Could you check a few things on this model? Use its own coordinates, in mm. Face numbers are marked on the shaded views. A direction names the side the tool comes from. Coordinates: 2 decimals unless noted, no trailing zeros. Write each loop counter-clockwise with the first axis right and the second up, starting at its lowest first coordinate (ties: lowest second). Pieces come first, ordered by that corner, then holes. Notation, with made-up numbers: M 23.5,39.5 L 55.5,39.5 A22 ccw 55.5,47.5 Z; hole C 9,79 d10. An arc over 180 degrees is marked long. Write item = value, one per line.
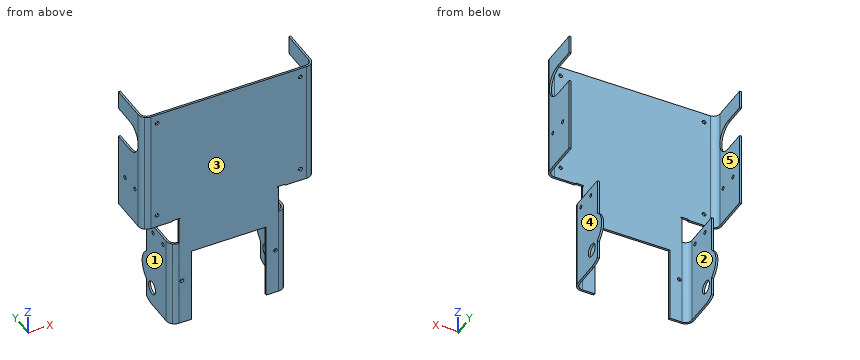
```python
from build123d import *

# Parameters (mm, degrees)
BOSS_EXTRUDE2_DEPTH     = 1.6
EDGE_FLANGE1_START      = -50
EDGE_FLANGE1_DEPTH      = 100
EDGE_FLANGE1_START_2    = -143
EDGE_FLANGE1_2_DEPTH    = 93.8
EDGE_FLANGE1_3_DEPTH    = 0.8
EDGE_FLANGE1_4_DEPTH    = 100
EDGE_FLANGE1_5_DEPTH    = 93
CUT_EXTRUDE1_START      = -71.5
CUT_EXTRUDE1_DEPTH      = 21.5
SKETCH24_R              = 15
BOSS_EXTRUDE3_DEPTH     = 1.6
BOSS_EXTRUDE4_START     = -1.6
SKETCH25_R              = 15
BOSS_EXTRUDE4_DEPTH     = 1.6
SKETCH26_R              = 5.25
CUT_EXTRUDE2_DEPTH      = 109.6
CUT_EXTRUDE3_DEPTH      = 1000
CUT_EXTRUDE4_DEPTH      = 188.95057861
CUT_EXTRUDE4_DEPTH_BACK = 188.95057861
SKETCH30_R              = 1.5
CUT_EXTRUDE5_DEPTH      = 204.484274577
CUT_EXTRUDE5_DEPTH_BACK = 204.484274577
SKETCH32_R              = 1.5
CUT_EXTRUDE6_DEPTH      = 54


# Read off the part's stored shape, not the designer's step: Edge-Flange1, Cut-Extrude1
with BuildPart() as part:
    # Sketch1 → Boss-Extrude2 (new body)
    with BuildSketch(Plane(origin=(0, 0, 0), x_dir=(1, 0, 0), z_dir=(0, 1, 0))):
        Polygon((45, 50), (45, 143), (30, 143), (30, 82), (-30, 82), (-30, 143), (-45, 143), (-45, 50), (-67.5, 50), (-67.5, -50), (67.5, -50), (67.5, 50), align=None)
    extrude(amount=BOSS_EXTRUDE2_DEPTH)

    # Edge-Flange1 outline → Edge-Flange1 (cut)
    with BuildSketch(Plane.XY.offset(EDGE_FLANGE1_START)):
        with BuildLine():
            Line((-67.5, 0), (-62.5, 0))
            ThreePointArc((-62.5, 0), (-64.797825059, 0.412916681), (-66.808131846, 1.6))
            Line((-66.808131846, 1.6), (-67.5, 1.6))
            Line((-67.5, 1.6), (-67.5, 0))
        make_face()
        with BuildLine():
            ThreePointArc((66.808131846, 1.6), (64.797825059, 0.412916681), (62.5, 0))
            Line((62.5, 0), (67.5, 0))
            Line((67.5, 0), (67.5, 1.6))
            Line((67.5, 1.6), (66.808131846, 1.6))
        make_face()
    extrude(amount=EDGE_FLANGE1_DEPTH, mode=Mode.SUBTRACT)

    # Edge-Flange1 2 outline → Edge-Flange1 2 (cut)
    with BuildSketch(Plane.XY.offset(EDGE_FLANGE1_START_2)):
        with BuildLine():
            Line((-45, 1.6), (-45, 0))
            Line((-45, 0), (-40, 0))
            ThreePointArc((-40, 0), (-42.297825059, 0.412916681), (-44.308131846, 1.6))
            Line((-44.308131846, 1.6), (-45, 1.6))
        make_face()
        with BuildLine():
            ThreePointArc((44.308131846, 1.6), (42.297825059, 0.412916681), (40, 0))
            Line((40, 0), (45, 0))
            Line((45, 0), (45, 1.6))
            Line((45, 1.6), (44.308131846, 1.6))
        make_face()
    extrude(amount=EDGE_FLANGE1_2_DEPTH, mode=Mode.SUBTRACT)

    # Edge-Flange1 3 outline → Edge-Flange1 3 (cut)
    with BuildSketch(Plane.XY.offset(EDGE_FLANGE1_START)):
        with BuildLine():
            ThreePointArc((-44.308131846, 1.6), (-42.297825059, 0.412916681), (-40, 0))
            Line((-40, 0), (-39.2, 0))
            Line((-39.2, 0), (-39.2, 1.6))
            Line((-39.2, 1.6), (-44.308131846, 1.6))
        make_face()
        with BuildLine():
            Line((39.2, 1.6), (39.2, 0))
            Line((39.2, 0), (40, 0))
            ThreePointArc((40, 0), (42.297825059, 0.412916681), (44.308131846, 1.6))
            Line((44.308131846, 1.6), (39.2, 1.6))
        make_face()
    extrude(amount=EDGE_FLANGE1_3_DEPTH, mode=Mode.SUBTRACT)

    # Edge-Flange1 4 outline → Edge-Flange1 4 (add)
    with BuildSketch(Plane.XY.offset(EDGE_FLANGE1_START)):
        with BuildLine():
            Line((-66.808131846, 1.6), (-62.5, 1.6))
            ThreePointArc((-62.5, 1.6), (-66.035533906, 3.064466094), (-67.5, 6.6))
            Line((-67.5, 6.6), (-67.5, 36.6))
            Line((-67.5, 36.6), (-69.1, 36.6))
            Line((-69.1, 36.6), (-69.1, 6.6))
            ThreePointArc((-69.1, 6.6), (-68.499736252, 3.84987911), (-66.808131846, 1.6))
        make_face()
        with BuildLine():
            ThreePointArc((67.5, 6.6), (66.035533906, 3.064466094), (62.5, 1.6))
            Line((62.5, 1.6), (66.808131846, 1.6))
            ThreePointArc((66.808131846, 1.6), (68.499736252, 3.84987911), (69.1, 6.6))
            Line((69.1, 6.6), (69.1, 36.6))
            Line((69.1, 36.6), (67.5, 36.6))
            Line((67.5, 36.6), (67.5, 6.6))
        make_face()
    extrude(amount=EDGE_FLANGE1_4_DEPTH)

    # Edge-Flange1 5 outline → Edge-Flange1 5 (add)
    with BuildSketch(Plane.XY.offset(EDGE_FLANGE1_START_2)):
        with BuildLine():
            ThreePointArc((-46.6, 6.6), (-45.999736252, 3.84987911), (-44.308131846, 1.6))
            Line((-44.308131846, 1.6), (-40, 1.6))
            ThreePointArc((-40, 1.6), (-43.535533906, 3.064466094), (-45, 6.6))
            Line((-45, 6.6), (-45, 36.6))
            Line((-45, 36.6), (-46.6, 36.6))
            Line((-46.6, 36.6), (-46.6, 6.6))
        make_face()
        with BuildLine():
            ThreePointArc((45, 6.6), (43.535533906, 3.064466094), (40, 1.6))
            Line((40, 1.6), (44.308131846, 1.6))
            ThreePointArc((44.308131846, 1.6), (45.999736252, 3.84987911), (46.6, 6.6))
            Line((46.6, 6.6), (46.6, 36.6))
            Line((46.6, 36.6), (45, 36.6))
            Line((45, 36.6), (45, 6.6))
        make_face()
    extrude(amount=EDGE_FLANGE1_5_DEPTH)

    # Cut-Extrude1 outline → Cut-Extrude1 (cut)
    with BuildSketch(Plane.XY.offset(CUT_EXTRUDE1_START)):
        with BuildLine():
            ThreePointArc((45, 6.6), (43.535533906, 3.064466094), (40, 1.6))
            Line((40, 1.6), (40, 0))
            ThreePointArc((40, 0), (44.666904756, 1.933095244), (46.6, 6.6))
            Line((46.6, 6.6), (46.6, 36.6))
            Line((46.6, 36.6), (45, 36.6))
            Line((45, 36.6), (45, 6.6))
        make_face()
        with BuildLine():
            ThreePointArc((-46.6, 6.6), (-44.666904756, 1.933095244), (-40, 0))
            Line((-40, 0), (-40, 1.6))
            ThreePointArc((-40, 1.6), (-43.535533906, 3.064466094), (-45, 6.6))
            Line((-45, 6.6), (-45, 36.6))
            Line((-45, 36.6), (-46.6, 36.6))
            Line((-46.6, 36.6), (-46.6, 6.6))
        make_face()
    extrude(amount=CUT_EXTRUDE1_DEPTH, mode=Mode.SUBTRACT)

    # Sketch24 → Boss-Extrude3 (add)
    with BuildSketch(Plane(origin=(46.6, 0, 0), x_dir=(0, 0, -1), z_dir=(1, 0, 0))):
        with Locations((113.002063462, 28.1)):
            Circle(SKETCH24_R)
    extrude(amount=-BOSS_EXTRUDE3_DEPTH)

    # Sketch25 → Boss-Extrude4 (add)
    with BuildSketch(Plane.ZY.offset(46.6).offset(BOSS_EXTRUDE4_START)):
        with Locations((-113.002063462, 28.1)):
            Circle(SKETCH25_R)
    extrude(amount=BOSS_EXTRUDE4_DEPTH)

    # Sketch26 → Cut-Extrude2 (cut)
    with BuildSketch(Plane(origin=(46.6, 0, 0), x_dir=(0, 0, -1), z_dir=(1, 0, 0))):
        with Locations(Location((128.002063462, 28.1, 0), (0, 0, 90))):
            Circle(SKETCH26_R)
        with BuildLine():
            Line((140.361270556, 36.6), (143, 36.6))
            Line((143, 36.6), (143, 28.348796314))
            ThreePointArc((143, 28.348796314), (142.289257641, 32.669035183), (140.361270556, 36.6))
        make_face()
    extrude(amount=-CUT_EXTRUDE2_DEPTH, mode=Mode.SUBTRACT)

    # Sketch27 → Cut-Extrude3 (cut)
    with BuildSketch(Plane(origin=(69.1, 0, 0), x_dir=(0, 0, -1), z_dir=(1, 0, 0))):
        with BuildLine():
            Line((-35.247936633, 19.100000095), (-35.247936633, 36.6))
            Line((-35.247936633, 36.6), (-10.247936633, 36.6))
            Line((-10.247936633, 36.6), (-10.247936633, 19.100000095))
            ThreePointArc((-10.247936633, 19.100000095), (-22.747936633, 6.600000095), (-35.247936633, 19.100000095))
        make_face()
    extrude(amount=-CUT_EXTRUDE3_DEPTH, mode=Mode.SUBTRACT)

    # Sketch30 → Cut-Extrude4 (cut, two sides: drawn at the far end of the back side and taken through both)
    with BuildSketch(Plane(origin=(-45, 0, 0), x_dir=(0, 0, -1), z_dir=(1, 0, 0)).offset(-CUT_EXTRUDE4_DEPTH_BACK)):
        with Locations(Location((78, 26.6, 0), (0, 0, 270))):
            Circle(SKETCH30_R)
        with Locations(Location((78, 11.6, 0), (0, 0, 270))):
            Circle(SKETCH30_R)
    extrude(amount=CUT_EXTRUDE4_DEPTH + CUT_EXTRUDE4_DEPTH_BACK, mode=Mode.SUBTRACT)

    # Sketch31 → Cut-Extrude5 (cut, two sides: drawn at the far end of the back side and taken through both)
    with BuildSketch(Plane(origin=(69.1, 0, 0), x_dir=(0, 0, -1), z_dir=(1, 0, 0)).offset(-CUT_EXTRUDE5_DEPTH_BACK)):
        with BuildLine():
            ThreePointArc((21.5, 26.6), (21.060660172, 27.660660172), (20, 28.1))
            Line((20, 28.1), (20, 25.1))
            ThreePointArc((20, 25.1), (21.060660172, 25.539339828), (21.5, 26.6))
        make_face()
        with BuildLine():
            Line((20, 25.1), (20, 28.1))
            ThreePointArc((20, 28.1), (18.5, 26.6), (20, 25.1))
        make_face()
        with BuildLine():
            ThreePointArc((21.5, 11.6), (21.060660172, 12.660660172), (20, 13.1))
            Line((20, 13.1), (20, 10.1))
            ThreePointArc((20, 10.1), (21.060660172, 10.539339828), (21.5, 11.6))
        make_face()
        with BuildLine():
            Line((20, 10.1), (20, 13.1))
            ThreePointArc((20, 13.1), (18.5, 11.6), (20, 10.1))
        make_face()
    extrude(amount=CUT_EXTRUDE5_DEPTH + CUT_EXTRUDE5_DEPTH_BACK, mode=Mode.SUBTRACT)

    # Sketch32 → Cut-Extrude6 (cut)
    with BuildSketch(Plane(origin=(0, 1.6, 0), x_dir=(1, 0, 0), z_dir=(0, 1, 0))):
        with Locations(Location((37.5, 105.642856368, 0), (0, 0, 270))):
            Circle(SKETCH32_R)
        with Locations(Location((57.5, 40.002063462, 0), (0, 0, 270))):
            Circle(SKETCH32_R)
        with Locations(Location((57.5, -42.497936538, 0), (0, 0, 270))):
            Circle(SKETCH32_R)
        with Locations(Location((-37.5, 105.642856368, 0), (0, 0, 90))):
            Circle(SKETCH32_R)
        with Locations(Location((-57.5, 40.002063462, 0), (0, 0, 90))):
            Circle(SKETCH32_R)
        with Locations(Location((-57.5, -42.497936538, 0), (0, 0, 90))):
            Circle(SKETCH32_R)
    extrude(amount=-CUT_EXTRUDE6_DEPTH, mode=Mode.SUBTRACT)


solid = part.part
```
Item 1: For the marked faces 4 and 5, which set-ups out of +Z, -Z, +X, -X, +Y, -Y let a thin tool reach every point of the face, with its end or its side?
Numbers:
face_4 = +Z, -Z, +X, +Y, -Y
face_5 = +Z, -Z, +Y
Item 2: If we mould it in two halves opening along X, with no side actions, what happens to the marked faces 1, 2 and 3? For each: pulls with the +X half, pulls with the -X half, needs draft (parallel to the pull), parting line crosses it, or undercut.
Numbers:
face_1 = pulls with the -X half
face_2 = undercut
face_3 = needs draft
Item 3: Imagine slicing it at B-B (y = 39). Write out the boundary of the cut face in (x, z), and give its area (3 significant figures).
Numbers:
outline = M -46.6,-123.31 L -45,-123.31 L -45,-102.7 L -46.6,-102.7 Z; M 45,-123.31 L 46.6,-123.31 L 46.6,-102.7 L 45,-102.7 Z
area = 66.0 mm²
Item 4: Imagine slicing it at D-D (x = 3). Write out the boundary of the cut face in (y, z), and give its area (3 significant figures).
Numbers:
outline = M 0,-82 L 1.6,-82 L 1.6,50 L 0,50 Z
area = 211 mm²
Item 5: Imagine slicing it at C-C (y = 16.5). Write out the boundary of the cut face in (x, z).
Numbers:
outline = M -69.1,-50 L -67.5,-50 L -67.5,10.52 L -69.1,10.52 Z; M -69.1,34.97 L -67.5,34.97 L -67.5,50 L -69.1,50 Z; M -46.6,-143 L -45,-143 L -45,-71.5 L -46.6,-71.5 Z; M 45,-143 L 46.6,-143 L 46.6,-71.5 L 45,-71.5 Z; M 67.5,-50 L 69.1,-50 L 69.1,10.52 L 67.5,10.52 Z; M 67.5,34.97 L 69.1,34.97 L 69.1,50 L 67.5,50 Z
Item 6: If I drill on line 1 along Z through (x, y) = (-57.5, 0.9); line 2 along X through (y, z) = (30, -94); line 3 along X through (y, z) = (16.5, -31), over which ranges is the centre line in solid material (lowest first)?
Numbers:
line_1 = -50 to -41.5, -38.5 to 41, 44 to 50
line_2 = -46.6 to -45, 45 to 46.6
line_3 = -69.1 to -67.5, 67.5 to 69.1
Item 7: I'm going to push flat-ended pins straight in: P1, Ø0.5, axis at y = 1, z = -61, coming from the -X side; P2, Ø1.3, axis at x = -46, z = -81, coming from the +Y side; P3, Ø12, axis at x = -57, y = 16, coming from the -Z side; P4, Ø1.5, axis at y = 5, z = -73.5, coming from the -X side. Where does each tip first touch, or does it pass through?
Numbers:
P1 = -40
P2 = 36.6
P3 = through
P4 = -46.55
Item 8: Imagine slicing it at A-A (z = -88.5). Write out the boundary of the cut face in (x, y), and give its area (3 significant figures).
Numbers:
outline = M -46.6,6.6 A6.6 ccw -40,0 L -30,0 L -30,1.6 L -40,1.6 A5 cw -45,6.6 L -45,36.6 L -46.6,36.6 Z; M 30,0 L 40,0 A6.6 ccw 46.6,6.6 L 46.6,36.6 L 45,36.6 L 45,6.6 A5 cw 40,1.6 L 30,1.6 Z
area = 157 mm²
